Here's how the part is built. I have some questions about the finished solid (model axes, mm). Face numbers are marked on the shaded views. A direction names the side the tool comes from. Round coordinates to 2 decimals unless told otherwise and drop trailing zeros. Loops run counter-clockwise (first coordinate to the right, second up) from the corner with the lowest first, then second, coordinate; pieces in that order, holes last. Notation, with made-up numbers: (-33.75, -9.75) -> (-19.75, -9.75) arc R21 cw to (-19.75, -2.75) -> close; hole circle Ø8 at (67, 18). An arc over 180 degrees is marked (long way). Use one line per item in the form item = value. Start each with the question number.
Item 1: If we section it at C-C (z = 10.75): Write out the boundary of the cut face in (x, y).
Item 2: If I drill on L1, parallel to X at y = 10.5, z = 2.5; L2, parallel to Y at x = 13, z = 6.25; L3, parallel to X at y = 6, z = 8, over which ranges is the centre line in solid material (lowest first)? Write a range as [from, to].
Item 3: I'm going to push flat-ended pins straight in: pin 1 Ø5 at (x, y) = (4, 16) entering from +Z; pin 2 Ø0.7 at (x, y) = (-15.5, -4.5) entering from +Z; pin 3 Ø0.6 at (x, y) = (-18, 10) entering from +Z. Where does each tip first touch, or does it pass through?
Item 4: If we section it at A-A (x = 23): Write out the boundary of the cut face in (y, z), then the cut area to 3 significant figures.
Item 5: If we section it at D-D (y = -4.5): Write out the boundary of the cut face in (x, z), then the cut area to 3 significant figures.
Item 6: For the marked faces 5 and 6, which set-ups out of +Z, -Z, +X, -X, +Y, -Y let a thin tool reach every point of the face, with its end or its side?
Item 7: Thinking about a two-plate mould opening in Y: for the marked faces 1, 2, 3 and 4, which applies, released by +Y, released by -Y, zero draft, split by the parting line, or undercut?
Item 8: If we section it at B-B (y = 20): Write out the boundary of the cut face in (x, z), then the cut area to 3 significant figures.
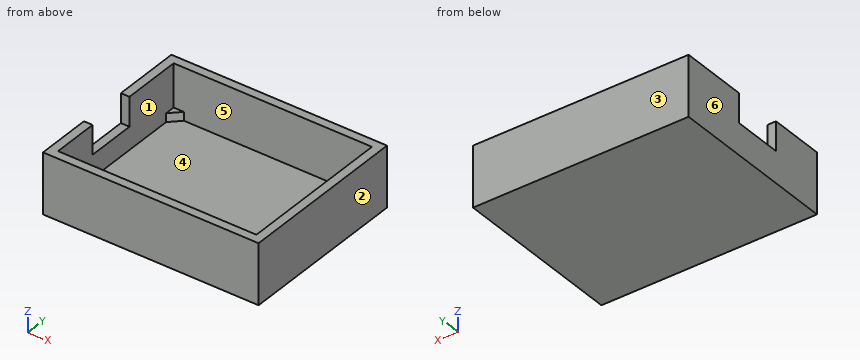
```python
from build123d import *

# Parameters (mm, degrees)
F1_DEPTH = 2
F2_DEPTH = 4
F0_W     = 50
F0_H     = 40
F3_DEPTH = 14
F4_W     = 11.5
F4_H     = 6.75
F5_DEPTH = 25


with BuildPart() as f1:
    # F0 (on Top) → F1 (new body)
    with BuildSketch(Plane.XY):
        Polygon((29.023395, 27.884433), (26.64808, 30.228337), (-14.601289, 30.228337), (-16.976605, 27.884433), (-16.976605, -3.427759), (-14.601289, -5.771663), (26.64808, -5.771663), (29.023395, -3.427759), align=None)
    extrude(amount=F1_DEPTH)

    # F0 (on Top) → F2 (join)
    with BuildSketch(Plane.XY):
        Polygon((-14.601289, -5.771663), (-16.976605, -3.427759), (-16.976605, -5.771663), align=None)
        Polygon((29.023395, -5.771663), (29.023395, -3.427759), (26.64808, -5.771663), align=None)
        Polygon((-16.976605, 27.884433), (-14.601289, 30.228337), (-16.976605, 30.228337), align=None)
        Polygon((29.023395, 27.884433), (29.023395, 30.228337), (26.64808, 30.228337), align=None)
    extrude(amount=F2_DEPTH)

    # F0 (on Top) → F3 (join)
    with BuildSketch(Plane.XY):
        with Locations((6.023395, 12.228337)):
            Rectangle(F0_W, F0_H)
        Polygon((26.64808, 30.228337), (29.023395, 30.228337), (29.023395, 27.884433), (29.023395, -3.427759), (29.023395, -5.771663), (26.64808, -5.771663), (-14.601289, -5.771663), (-16.976605, -5.771663), (-16.976605, -3.427759), (-16.976605, 27.884433), (-16.976605, 30.228337), (-14.601289, 30.228337), align=None, mode=Mode.SUBTRACT)
    extrude(amount=F3_DEPTH)

    # F4 (on face) → F5 (cut)
    with BuildSketch(Plane(origin=(-18.976605, 0, 0), x_dir=(0, -1, 0), z_dir=(-1, 0, 0))):
        with Locations((-10.728337, 10.625)):
            Rectangle(F4_W, F4_H)
    extrude(amount=-F5_DEPTH, mode=Mode.SUBTRACT)


solid = f1.part
```
Values found:
q1.outline = (-18.98, -7.77) -> (31.02, -7.77) -> (31.02, 32.23) -> (-18.98, 32.23) -> (-18.98, 16.48) -> (-16.98, 16.48) -> (-16.98, 30.23) -> (29.02, 30.23) -> (29.02, -5.77) -> (-16.98, -5.77) -> (-16.98, 4.98) -> (-18.98, 4.98) -> close
q2.L1 = [-18.98, -16.98], [29.02, 31.02]
q2.L2 = [-7.77, -5.77], [30.23, 32.23]
q2.L3 = [29.02, 31.02]
q3.pin_1 = 2
q3.pin_2 = 4
q3.pin_3 = 7.25
q4.outline = (-7.77, 0) -> (32.23, 0) -> (32.23, 14) -> (30.23, 14) -> (30.23, 2) -> (-5.77, 2) -> (-5.77, 14) -> (-7.77, 14) -> close
q4.area = 128 mm2
q5.outline = (-18.98, 0) -> (31.02, 0) -> (31.02, 14) -> (29.02, 14) -> (29.02, 4) -> (27.94, 4) -> (27.94, 2) -> (-15.89, 2) -> (-15.89, 4) -> (-16.98, 4) -> (-16.98, 14) -> (-18.98, 14) -> close
q5.area = 152 mm2
q6.face_5 = +Z
q6.face_6 = +Z, -Z, -X, +Y, -Y
q7.face_1 = undercut
q7.face_2 = zero draft
q7.face_3 = released by +Y
q7.face_4 = undercut
q8.outline = (-18.98, 0) -> (31.02, 0) -> (31.02, 14) -> (29.02, 14) -> (29.02, 2) -> (-16.98, 2) -> (-16.98, 14) -> (-18.98, 14) -> close
q8.area = 148 mm2
